```python
from build123d import *

# Parameters (mm, degrees)
MAIN_SKETCH_R     = 4
MAIN_SKETCH_R_2   = 1.65
WASHER_MAIN_DEPTH = 0.8
EDGE_FILLETS_R    = 0.2


with BuildPart() as part:
    # Main Sketch → Washer Main (new body)
    with BuildSketch(Plane(origin=(0, 0, 0), x_dir=(1, 0, 0), z_dir=(0, 1, 0))):
        with Locations(Location((0, 0, 0), (0, 0, 270))):
            Circle(MAIN_SKETCH_R)
        with Locations(Location((0, 0, 0), (0, 0, 270))):
            Circle(MAIN_SKETCH_R_2, mode=Mode.SUBTRACT)
    extrude(amount=WASHER_MAIN_DEPTH)

    # Edge Fillets
    edge_fillets_edges = [part.edges().sort_by_distance(p)[0] for p in [
        (0, 0, -4),
        (0, 0.8, -4),
        (0, 0, -1.65),
        (0, 0.8, -1.65),
    ]]
    fillet(edge_fillets_edges, radius=EDGE_FILLETS_R)


solid = part.part
```
Source: CAD feature listing. Evaluate the final solid. Frame: model axes, mm. Coordinates: 2 decimals unless noted, no trailing zeros. Order: outer loops, then holes, each group sorted by start corner. A loop starts at its lowest first (then second) coordinate and runs counter-clockwise, first axis right, second up. Notation, with made-up numbers: (-39, 78) - (-16, 78) arc R22 ccw to (-16, 115) - close; hole circle Ø9 at (46, -5). An arc over 180 degrees is marked (long way). One line per item, written item: value.
1) Cut plane C-C on y = 0.5. Output: boundary loops of the cut face in (x, z).
Computed values:
outline: circle Ø8 at (0, 0); hole circle Ø3.3 at (0, 0)
2) Ray query, line 1 (X direction, y = 0.4, z = 0); line 2 (X direction, y = 0.65, z = 1.5); line 3 (Z direction, x = -0.75, y = 0.1). Return the intervals inside material, ascending. Write a range as [from, to].
Computed values:
line 1: x = [-4, -1.65], [1.65, 4]
line 2: x = [-3.7, -0.7], [0.7, 3.7]
line 3: z = [-3.9, -1.5], [1.5, 3.9]
3) Contact query for flat-ended pins moving along their axis: pin 1 (3 mm diameter, centred on x = 0, z = 0, fed in from -Y); pin 2 (1 mm diameter, centred on x = 0, z = 3, fed in from -Y). Output: stop coordinate, or through.
Computed values:
pin 1: passes through
pin 2: stops at y = 0
4) Cut plane B-B on z = 0. Output: boundary loops of the cut face in (x, y), plus the area to 3 significant figures.
Computed values:
outline: (-4, 0.2) arc R0.2 ccw to (-3.8, 0) - (-1.85, 0) arc R0.2 ccw to (-1.65, 0.2) - (-1.65, 0.6) arc R0.2 ccw to (-1.85, 0.8) - (-3.8, 0.8) arc R0.2 ccw to (-4, 0.6) - close; (1.65, 0.2) arc R0.2 ccw to (1.85, 0) - (3.8, 0) arc R0.2 ccw to (4, 0.2) - (4, 0.6) arc R0.2 ccw to (3.8, 0.8) - (1.85, 0.8) arc R0.2 ccw to (1.65, 0.6) - close
area: 3.69 mm^2
5) Cut plane A-A on x = 0. Output: boundary loops of the cut face in (y, z), plus the area to 3 significant figures.
Computed values:
outline: (0, -3.8) arc R0.2 ccw to (0.2, -4) - (0.6, -4) arc R0.2 ccw to (0.8, -3.8) - (0.8, -1.85) arc R0.2 ccw to (0.6, -1.65) - (0.2, -1.65) arc R0.2 ccw to (0, -1.85) - close; (0, 1.85) arc R0.2 ccw to (0.2, 1.65) - (0.6, 1.65) arc R0.2 ccw to (0.8, 1.85) - (0.8, 3.8) arc R0.2 ccw to (0.6, 4) - (0.2, 4) arc R0.2 ccw to (0, 3.8) - close
area: 3.69 mm^2
6) Mould query, pull axis Z, two halves, no side actions, for faces 1 (the face through (-3.905, 0.397, -0.867)), 2 (the face through (1, 0, 2)), 3 (the face through (-1, 0.4, -1.31)). Classes: released by +Z, released by -Z, zero draft, split by the parting line, or undercut.
Computed values:
face 1: split by the parting line
face 2: zero draft
face 3: undercut
